The figure shows three views and two pictorial views of one solid part (mm, origin at its lowest corner). Answer the questions. A direction names the side the tool comes from. Coordinates: 2 decimals unless noted, no trailing zeros. Loops run counter-clockwise (first coordinate to the right, second up) from the corner with the lowest first, then second, coordinate; pieces in that order, holes last.
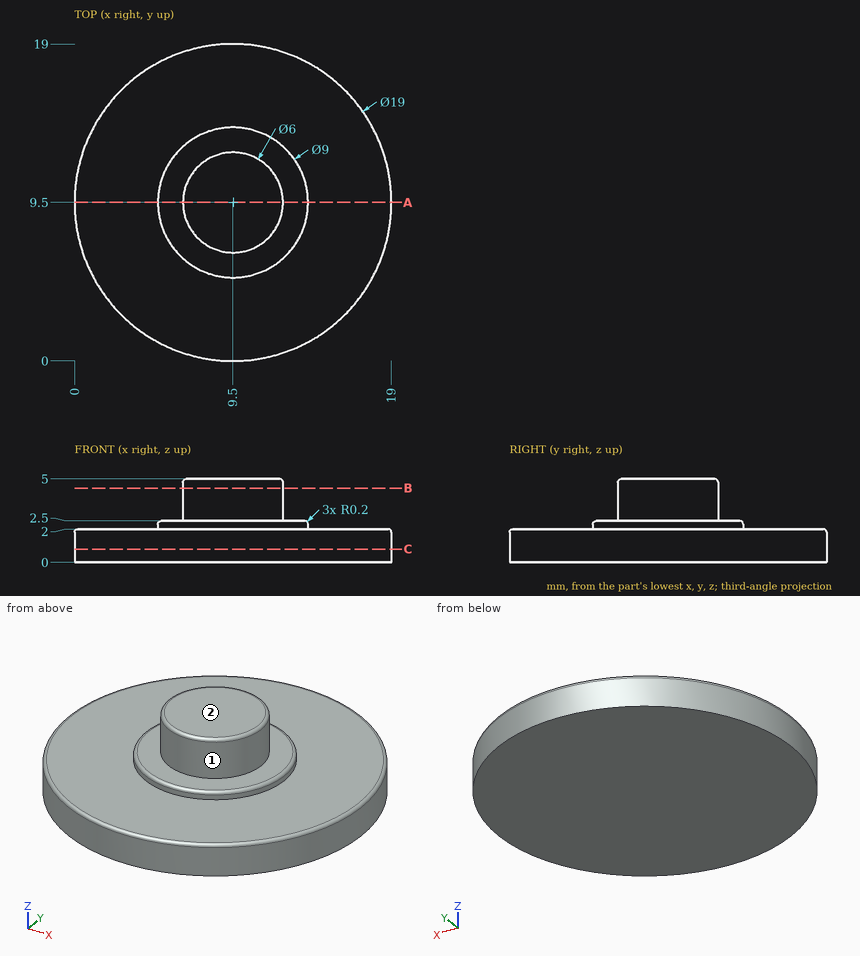
1. For the marked faces 1 and 2, determine the directions among +Z, -Z, +X, -X, +Y, -Y from which every point of the face is accessible in a straight line to the end or side of a thin tool.
2. Straight lines are drawn through the part: probe 1 along Z at (x, y) = (7.25, 17.5); probe 2 along Z at (x, y) = (9, 5.25); probe 3 along Y at (x, z) = (3.5, 1.05). For each, find the intervals that lie inside material, in ascending order.
3. A cutting plane is placed at B-B, the plane z = 4.45. Give the vertices of the cut face in (x, y).
4. A cutting plane is placed at C-C, the plane z = 0.8. Give the vertices of the cut face in (x, y), then the cut area to 3 significant figures.
5. A cutting plane is placed at A-A, the plane y = 9.5. Give the vertices of the cut face in (x, z).
6. This flat-tipped pin is pushed along its axis until it touches: P1, Ø1.5, axis at x = 5.5, z = 2.5, coming from the +Y side. Where does it stop, or does it pass through?
Answers below:
1. face 1: +Z
1. face 2: +Z, +X, -X, +Y, -Y
2. probe 1: z = 0 to 2
2. probe 2: z = 0 to 2.5
2. probe 3: y = 2.13 to 16.87
3. outline: circle Ø6 at (9.5, 9.5)
4. outline: circle Ø19 at (9.5, 9.5)
4. area: 284 mm2
5. outline: (0, 0) - (19, 0) - (19, 1.8) arc R0.2 ccw to (18.8, 2) - (14, 2) - (14, 2.3) arc R0.2 ccw to (13.8, 2.5) - (12.5, 2.5) - (12.5, 4.8) arc R0.2 ccw to (12.3, 5) - (6.7, 5) arc R0.2 ccw to (6.5, 4.8) - (6.5, 2.5) - (5.2, 2.5) arc R0.2 ccw to (5, 2.3) - (5, 2) - (0.2, 2) arc R0.2 ccw to (0, 1.8) - close
6. P1: stops at y = 18.28
